Geometry: final body of the model. Coordinates: model frame, mm. Round coordinates to 2 decimals unless told otherwise and drop trailing zeros. Loops run counter-clockwise (first coordinate to the right, second up) from the corner with the lowest first, then second, coordinate; pieces in that order, holes last. Notation, with made-up numbers: (16.25, -6) -> (60.25, -6) arc R25 cw to (60.25, 6) -> close; hole circle Ø3 at (66, -0.5). An arc over 180 degrees is marked (long way). Answer in a Markdown table with one row per item.
Autodesk Inventor part; units mm, degrees
ref_plane "YZ Plane" through (0, 0, 0) normal (1, 0, 0) x (0, 1, 0)
ref_plane "XZ Plane" through (0, 0, 0) normal (0, 1, 0) x (-1, 0, 0)
ref_plane "XY Plane" through (0, 0, 0) normal (0, 0, 1) x (1, 0, 0)
sketch "Sketch1" plane through (0, 0, 0) normal (0, 0, 1) x (1, 0, 0)
  line L0 (-91.239, 32) -> (-91.239, 35)
  line L1 (51.239, 32) -> (51.239, 35)
  line L2 (51.239, -41) -> (51.239, -38)
  line L3 (-91.239, 35) -> (51.239, 35)
  line L4 (51.239, 35) -> (51.239, -41)
  line L5 (51.239, -41) -> (-91.239, -41)
  line L6 (-91.239, -41) -> (-91.239, 35)
  point P0 (0, 0)
extrude "Extrusion1" add sketch "Sketch1" against normal blind 3
sketch "Sketch2" plane through (0, 0, 0) normal (0, 0, 1) x (1, 0, 0)
  line L0 (-80, 35) -> (-80, 32)
  line L1 (-80, 32) -> (-50, 32)
  line L2 (-50, 32) -> (-50, 35)
  line L3 (-80, 35) -> (-50, 35)
  line L4 (-10, 32) -> (-10, 35)
  line L5 (-30, 35) -> (-10, 35)
  line L6 (-30, 35) -> (-30, 32)
  line L7 (-30, 32) -> (-10, 32)
  line L8 (-50, 0) -> (-70, 0)
  line L9 (-70, 0) -> (-70, -3)
  line L10 (-70, -3) -> (-50, -3)
  line L11 (-50, 0) -> (-50, -3)
  line L12 (-30, 0) -> (-40, 0)
  line L13 (-40, 0) -> (-40, -3)
  line L14 (-40, -3) -> (-30, -3)
  line L15 (-30, 0) -> (-30, -3)
  line L16 (-80, -28) -> (-80, -18)
  line L17 (-80, -28) -> (-77, -28)
  line L18 (-77, -18) -> (-77, -28)
  line L19 (-80, -18) -> (-77, -18)
  line L20 (-80, 2) -> (-80, 22)
  line L21 (-80, 2) -> (-77, 2)
  line L22 (-77, 22) -> (-77, 2)
  line L23 (-80, 22) -> (-77, 22)
  line L24 (-80, -41) -> (-80, -38)
  line L25 (-91.239, -38) -> (-80, -38)
  line L26 (-91.239, -41) -> (-91.239, -38)
  line L27 (-91.239, -41) -> (-80, -41)
  line L28 (-40, -41) -> (-40, -38)
  line L29 (-60, -38) -> (-40, -38)
  line L30 (-60, -38) -> (-60, -41)
  line L31 (-60, -41) -> (-40, -41)
  line L32 (-10, -41) -> (-10, -38)
  line L33 (-30, -38) -> (-10, -38)
  line L34 (-30, -38) -> (-30, -41)
  line L35 (-30, -41) -> (-10, -41)
  point P0 (0, 0)
extrude "Extrusion2" cut sketch "Sketch2" against normal blind 3 contours L3 L2 L1 L0 | L7 L6 L5 L4 | L11 L10 L9 L8 | L15 L14 L13 L12 | L20 L23 L22 L21 | L27 L26 L25 L24 | L31 L30 L29 L28 | L35 L34 L33 L32
sketch "Sketch3" plane through (0, 0, 0) normal (0, 0, 1) x (1, 0, 0)
  line L0 (-90, 32) -> (-90, 35)
  line L1 (-91.239, 35) -> (-90, 35)
  line L2 (-91.239, 32) -> (-91.239, 35)
  line L3 (-91.239, 32) -> (-90, 32)
  line L4 (-87.5, -3) -> (-82.5, -3)
  line L5 (-87.5, -6) -> (-82.5, -6)
  line L6 (-82.5, -6) -> (-82.5, -3)
  line L7 (-87.5, -6) -> (-87.5, -3)
  line L8 (-77, -18) -> (-77, -28)
  line L9 (-80, -28) -> (-80, -18)
  line L10 (-80, -18) -> (-77, -18)
  line L11 (-80, -28) -> (-77, -28)
  line L12 (-55, -10.5) -> (-55, -30.5)
  line L13 (-55, -10.5) -> (-58, -10.5)
  line L14 (-58, -30.5) -> (-58, -10.5)
  line L15 (-55, -30.5) -> (-58, -30.5)
  point P0 (0, 0)
extrude "Extrusion3" cut sketch "Sketch3" against normal blind 3
ref_plane "Work Plane1" through (-20, -41, 0) normal (1, 0, 0) x (0, 0, -1)
mirror "Mirror1" about plane through (-20, -41, 0) normal (1, 0, 0) of "Extrusion3", "Extrusion2"
properties part number "Frount"
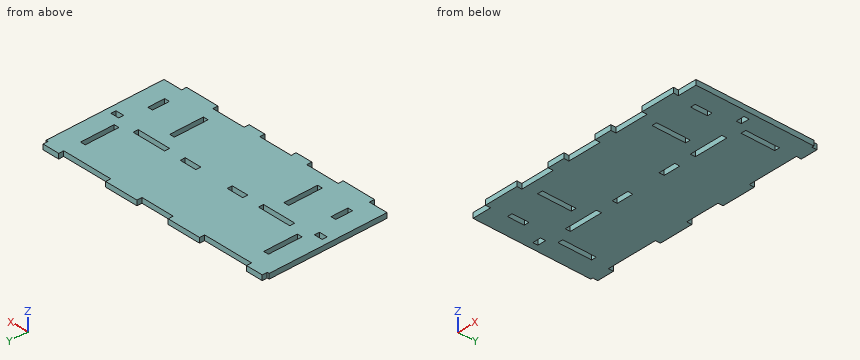
Item 1: Section query B-B, the plane x = 13. Output: boundary loops of the cut face in (y, z).
Ans:
| item | result |
|---|---|
| outline | (-38, -3) -> (-3, -3) -> (-3, 0) -> (-38, 0) -> close; (0, -3) -> (32, -3) -> (32, 0) -> (0, 0) -> close |
Item 2: Section query C-C, the plane x = 38.5. Output: boundary loops of the cut face in (y, z), and give its area (3 significant figures).
Ans:
| item | result |
|---|---|
| outline | (-41, -3) -> (-28, -3) -> (-28, 0) -> (-41, 0) -> close; (-18, -3) -> (2, -3) -> (2, 0) -> (-18, 0) -> close; (22, -3) -> (32, -3) -> (32, 0) -> (22, 0) -> close |
| area | 129 mm2 |
Item 3: Section query D-D, the plane z = -2. State how many separate pieces and enclosed holes the cut face has, and give its area (3 significant figures).
Ans:
| item | result |
|---|---|
| separate pieces | 1 |
| enclosed holes | 12 |
| area | 9,820 mm2 |
Item 4: Ray query, L1, parallel to Y at x = 38.5, z = -1.15; L2, parallel to X at y = -17, z = -2.1; L3, parallel to X at y = 10.5, z = -0.9. Return the intervals inside material, ascending.
Ans:
| item | result |
|---|---|
| L1 | -41 to -28, -18 to 2, 22 to 32 |
| L2 | -91.24 to -58, -55 to 15, 18 to 51.24 |
| L3 | -91.24 to -80, -77 to 37, 40 to 51.24 |
Item 5: First-contact query: P1, Ø1, axis at x = -73.5, z = -2.5, coming from the +Y side; P2, Ø1.5, axis at x = 17.5, z = -2, coming from the -Y side; P3, Ø1.5, axis at y = 33.5, z = -2, coming from the +X side. Flat tips, straight axial feed; report the tip coordinate or a pass-through.
Ans:
| item | result |
|---|---|
| P1 | y = 32 |
| P2 | y = -38 |
| P3 | x = 50 |
Item 6: Section query A-A, the plane y = -24. Output: boundary loops of the cut face in (x, z), and give its area (3 significant figures).
Ans:
| item | result |
|---|---|
| outline | (-91.24, -3) -> (-80, -3) -> (-80, 0) -> (-91.24, 0) -> close; (-77, -3) -> (-58, -3) -> (-58, 0) -> (-77, 0) -> close; (-55, -3) -> (15, -3) -> (15, 0) -> (-55, 0) -> close; (18, -3) -> (37, -3) -> (37, 0) -> (18, 0) -> close; (40, -3) -> (51.24, -3) -> (51.24, 0) -> (40, 0) -> close |
| area | 391 mm2 |
